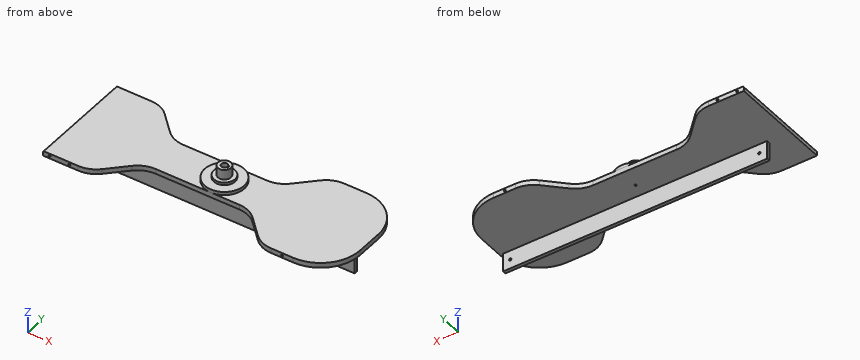
from build123d import *

# Parameters (mm, degrees)
BOSS_EXTRUDE1_DEPTH        = 9.525
SKETCH6_W                  = 509.27
SKETCH6_H                  = 6.35
BOSS_EXTRUDE3_DEPTH        = 35.56
SKETCH7_R                  = 2.286
CUT_EXTRUDE4_DEPTH         = 575.152378381
F_10_32_TAPPED_HOLE1_D     = 4.0386
F_10_32_TAPPED_HOLE1_DEPTH = 13.716
F_10_32_TAPPED_HOLE1_TIP   = 1.213317848
F_10_32_TAPPED_HOLE2_D     = 4.0386
F_10_32_TAPPED_HOLE2_DEPTH = 13.716
F_10_32_TAPPED_HOLE2_TIP   = 1.213317848
SKETCH12_R                 = 38.1
BOSS_EXTRUDE4_DEPTH        = 6.35
SKETCH13_R                 = 20.447
BOSS_EXTRUDE5_DEPTH        = 5.08
SKETCH14_R                 = 12.573
BOSS_EXTRUDE6_DEPTH        = 19.05
CUT_EXTRUDE5_DEPTH         = 19.05
FILLET1_R                  = 2.54
F_10_32_TAPPED_HOLE3_D     = 4.0386


with BuildPart() as part:
    # Sketch1 → Boss-Extrude1 (new body)
    with BuildSketch(Plane.XY):
        with BuildLine():
            Line((103.778975516, 188.321024484), (137.521024484, 154.578975516))
            ThreePointArc((137.521024484, 154.578975516), (154.001730604, 143.566919748), (173.442048969, 139.7))
            Line((173.442048969, 139.7), (334.557951031, 139.7))
            ThreePointArc((334.557951031, 139.7), (353.998269396, 143.566919748), (370.478975516, 154.578975516))
            Line((370.478975516, 154.578975516), (404.221024484, 188.321024484))
            ThreePointArc((404.221024484, 188.321024484), (420.701730604, 199.333080252), (440.142048969, 203.2))
            Line((440.142048969, 203.2), (482.6, 203.2))
            ThreePointArc((482.6, 203.2), (536.481536726, 180.881536726), (558.8, 127))
            Line((558.8, 127), (558.8, 76.2))
            ThreePointArc((558.8, 76.2), (536.481536726, 22.318463274), (482.6, 0))
            Line((482.6, 0), (440.142048969, 0))
            ThreePointArc((440.142048969, 0), (420.701730604, 3.866919748), (404.221024484, 14.878975516))
            Line((404.221024484, 14.878975516), (370.478975516, 48.621024484))
            ThreePointArc((370.478975516, 48.621024484), (353.998269396, 59.633080252), (334.557951031, 63.5))
            Line((334.557951031, 63.5), (173.442048969, 63.5))
            ThreePointArc((173.442048969, 63.5), (154.001730604, 59.633080252), (137.521024484, 48.621024484))
            Line((137.521024484, 48.621024484), (103.778975516, 14.878975516))
            ThreePointArc((103.778975516, 14.878975516), (87.298269396, 3.866919748), (67.857951031, 0))
            Line((67.857951031, 0), (0, 0))
            Line((0, 0), (0, 203.2))
            Line((0, 203.2), (67.857951031, 203.2))
            ThreePointArc((67.857951031, 203.2), (87.298269396, 199.333080252), (103.778975516, 188.321024484))
        make_face()
    extrude(amount=BOSS_EXTRUDE1_DEPTH)

    # Sketch6 → Boss-Extrude3 (add)
    with BuildSketch(Plane(origin=(0, 0, 0), x_dir=(-1, 0, 0), z_dir=(0, 0, -1))):
        with Locations((-297.815, 73.025)):
            Rectangle(SKETCH6_W, SKETCH6_H)
    extrude(amount=BOSS_EXTRUDE3_DEPTH)

    # Sketch7 → Cut-Extrude4 (cut, through all)
    with BuildSketch(Plane(origin=(0, 76.2, 0), x_dir=(1, 0, 0), z_dir=(0, 1, 0))):
        with Locations(Location((58.166, 17.78, 0), (0, 0, 270))):
            Circle(SKETCH7_R)
        with Locations(Location((538.734, 17.78, 0), (0, 0, 270))):
            Circle(SKETCH7_R)
    extrude(amount=-CUT_EXTRUDE4_DEPTH, mode=Mode.SUBTRACT)

    # #10-32 Tapped Hole1
    with Locations(Plane(origin=(0, 203.2, 0), x_dir=(-1, 0, 0), z_dir=(0, 1, 0))):
        with Locations((-12.7, 4.7625), (-50.8, 4.7625), (-461.01, 4.7625)):
            Hole(F_10_32_TAPPED_HOLE1_D / 2, depth=F_10_32_TAPPED_HOLE1_DEPTH)
            with Locations((0, 0, -(F_10_32_TAPPED_HOLE1_DEPTH + F_10_32_TAPPED_HOLE1_TIP / 2))):  # 118° drill point
                Cone(0, F_10_32_TAPPED_HOLE1_D / 2, F_10_32_TAPPED_HOLE1_TIP, mode=Mode.SUBTRACT)

    # #10-32 Tapped Hole2
    with Locations(Plane.XZ):
        with Locations((12.7, 4.7625), (50.8, 4.7625), (461.01, 4.7625)):
            Hole(F_10_32_TAPPED_HOLE2_D / 2, depth=F_10_32_TAPPED_HOLE2_DEPTH)
            with Locations((0, 0, -(F_10_32_TAPPED_HOLE2_DEPTH + F_10_32_TAPPED_HOLE2_TIP / 2))):  # 118° drill point
                Cone(0, F_10_32_TAPPED_HOLE2_D / 2, F_10_32_TAPPED_HOLE2_TIP, mode=Mode.SUBTRACT)

    # Sketch12 → Boss-Extrude4 (add)
    with BuildSketch(Plane.XY.offset(9.525)):
        with Locations(Location((279.4, 101.6, 0), (0, 0, 270))):
            Circle(SKETCH12_R)
    extrude(amount=BOSS_EXTRUDE4_DEPTH)

    # Sketch13 → Boss-Extrude5 (add)
    with BuildSketch(Plane.XY.offset(15.875)):
        with Locations((279.4, 101.6)):
            Circle(SKETCH13_R)
    extrude(amount=BOSS_EXTRUDE5_DEPTH)

    # Sketch14 → Boss-Extrude6 (add)
    with BuildSketch(Plane.XY.offset(20.955)):
        with Locations(Location((279.4, 101.6, 0), (0, 0, 180))):
            Circle(SKETCH14_R)
    extrude(amount=BOSS_EXTRUDE6_DEPTH)

    # Sketch15 → Cut-Extrude5 (cut)
    with BuildSketch(Plane.XY.offset(40.005)):
        with BuildLine():
            Line((287.401, 103.7082), (287.401, 99.4918))
            Line((287.401, 99.4918), (285.294277832, 99.4918))
            ThreePointArc((285.294277832, 99.4918), (285.151947147, 99.448175797), (285.058506719, 99.332288))
            ThreePointArc((285.058506719, 99.332288), (273.304, 101.6), (285.058506719, 103.867712))
            ThreePointArc((285.058506719, 103.867712), (285.151947147, 103.751824203), (285.294277832, 103.7082))
            Line((285.294277832, 103.7082), (287.401, 103.7082))
        make_face()
    extrude(amount=-CUT_EXTRUDE5_DEPTH, mode=Mode.SUBTRACT)

    # Fillet1
    fillet1_edges = [part.edges().sort_by_distance(p)[0] for p in [
        (0, 101.6, 9.525),
    ]]
    fillet(fillet1_edges, radius=FILLET1_R)

    # #10-32 Tapped Hole3 (through all)
    with Locations(Plane(origin=(279.4, 101.6, 20.955), x_dir=(1, 0, 0), z_dir=(0, 0, 1))):
        with Locations((0, 0)):
            Hole(F_10_32_TAPPED_HOLE3_D / 2)


solid = part.part
CAD build for the part. Positions are in the model's coordinates, mm. Round coordinates to 2 decimals unless told otherwise and drop trailing zeros. Write each loop counter-clockwise with the first axis right and the second up, starting at its lowest first coordinate (ties: lowest second). Pieces come first, ordered by that corner, then holes. Notation, with made-up numbers: M 84.5,-15 L 98.5,-15 A10 cw 98.5,-11 Z; hole C 8,9 d8. An arc over 180 degrees is marked long. Put each result on its own line as item: value. Start each with the question number.
1) Drill centre lines: probe 1 along Z at (x, y) = (12.7, 10.75) (3 decimals); probe 2 along Y at (x, z) = (279, 32); probe 3 along X at (y, z) = (101.6, 33). Where is each one in solid material? Low to high. Write a range as [from, to].
2) Pin check, flat tips, straight feed: pin 1 Ø3 at (x, y) = (424, 85) entering from -Z; pin 2 Ø4.5 at (y, z) = (101, 27) entering from -X; pin 3 Ø1.7 at (x, z) = (286.5, 30) entering from -Y; pin 4 Ø2.5 at (x, y) = (279.4, 101.6) entering from -Z. Stop position of each tip, or through.
3) Saw through at A-A, the plane y = 175.5. Write the cut outline in (x, z) (3 decimals).
Resolved:
1. probe 1: [0, 2.743], [6.782, 9.525]
1. probe 2: [89.03, 95.52], [107.68, 114.17]
1. probe 3: [266.83, 273.3], [287.4, 291.97]
2. pin 1: z = 0
2. pin 2: x = 266.83
2. pin 3: y = 90.69
2. pin 4: through
3. outline: M 0,0 L 116.6,0 L 116.6,9.525 L 2.54,9.525 A2.54 ccw 0,6.985 Z; M 391.4,0 L 541.372,0 L 541.372,9.525 L 391.4,9.525 Z
